Build history of the part. All positions in model axes, mm. A direction names the side the tool comes from. Round coordinates to 2 decimals unless told otherwise and drop trailing zeros. Order: outer loops, then holes, each group sorted by start corner. A loop starts at its lowest first (then second) coordinate and runs counter-clockwise, first axis right, second up. Notation, with made-up numbers: (49.25, 88) - (57.25, 88) arc R11 ccw to (57.25, 93) - close; hole circle Ø11 at (-17, 44). An arc over 180 degrees is marked (long way). One line per question, with ' | ' between items. Start each with the question number.
Autodesk Inventor part; units mm, degrees
ref_plane "YZ Plane" through (0, 0, 0) normal (1, 0, 0) x (0, 1, 0)
ref_plane "XZ Plane" through (0, 0, 0) normal (0, 1, 0) x (-1, 0, 0)
ref_plane "XY Plane" through (0, 0, 0) normal (0, 0, 1) x (1, 0, 0)
sketch "スケッチ1" plane through (0, 0, 0) normal (0, 1, 0) x (-1, 0, 0)
  line L0 (-15, -7.5) -> (15, -7.5)
  line L1 (15, -7.5) -> (15, 7.5)
  line L2 (15, 7.5) -> (-15, 7.5)
  line L3 (-15, 7.5) -> (-15, -7.5)
  line L4 (-15, -7.5) -> (15, 7.5) construction
  line L5 (15, -7.5) -> (-15, 7.5) construction
  point P0 (0, 0)
  dimension "d0" = 30
  dimension "d1" = 15
extrude "押し出し1" add sketch "スケッチ1" along normal mid plane 10
sketch "スケッチ2" plane through (0, 0, 0) normal (0, 1, 0) x (-1, 0, 0)
  line L0 (15, 7.5) -> (-15, 7.5)
  line L1 (10, 7.5) -> (-15, 7.5)
  line L2 (-15, 7.5) -> (-15, 1.5)
  line L3 (-15, 1.5) -> (10, 1.5)
  line L4 (10, 1.5) -> (10, 7.5)
  point P0 (0, 0)
  dimension "d4" = 25
  dimension "d5" = 6
  dimension "d6" = 5
extrude "押し出し2" cut sketch "スケッチ2" along normal mid plane 10
sketch "スケッチ3" plane through (0, 0, 0) normal (0, 1, 0) x (-1, 0, 0)
  line L0 (15, -7.5) -> (-15, -7.5)
  line L1 (-15, -7.5) -> (10, -7.5)
  line L2 (10, -7.5) -> (10, -1.5)
  line L3 (10, -1.5) -> (-15, -1.5)
  line L4 (-15, -1.5) -> (-15, -7.5)
  point P0 (0, 0)
  dimension "d9" = 25
  dimension "d10" = 6
extrude "押し出し3" cut sketch "スケッチ3" along normal mid plane 10
sketch "スケッチ4" plane through (0, 0, 0) normal (1, 0, 0) x (0, 1, 0)
  line L0 (2, 7.5) -> (-2, 7.5)
  line L1 (-2, 7.5) -> (-2, 2.5)
  line L2 (-2, 2.5) -> (2, 2.5)
  line L3 (2, 2.5) -> (2, 7.5)
  point P0 (0, 0)
  dimension "d13" = 4
  dimension "d14" = 5
  dimension "d15" = 2
  dimension "d16" = 7.5
extrude "押し出し4" cut sketch "スケッチ4" against normal blind 15
sketch "スケッチ6" plane through (0, 5, 0) normal (0, 1, 0) x (1, 0, 0)
  circle A0 centre (-12.5, -5) radius 1.25
  line L0 (-15, -7.5) -> (-10, -7.5)
  point P0 (0, 0)
  dimension "d23" = 2.5
  dimension "d24" = 2.5
extrude "押し出し5" cut sketch "スケッチ6" against normal blind 15
sketch "スケッチ7" plane through (0, 5, 0) normal (0, 1, 0) x (1, 0, 0)
  circle A0 centre (-12.5, 5) radius 1.25
  line L0 (-10, 7.5) -> (-15, 7.5)
  line L1 (-15, 7.5) -> (-15, -7.5)
  point P0 (0, 0)
  dimension "d27" = 2.5
  dimension "d28" = 2.5
extrude "押し出し6" cut sketch "スケッチ7" against normal blind 15
sketch "スケッチ8" plane through (-10, -5, -1.5) normal (1, 0, 0) x (0, 0, -1)
  line L0 (1, 7) -> (6, 7)
  line L1 (6, 7) -> (6, 3)
  line L2 (6, 3) -> (1, 3)
  line L3 (1, 3) -> (1, 7)
  point P0 (-1.5, 5)
  dimension "d32" = 5
  dimension "d33" = 4
  dimension "d34" = 7.5
  dimension "d35" = 2
extrude "押し出し7" cut sketch "スケッチ8" against normal blind 15
properties part number "promo_hold"
Item 1: Slice it at A-A (z = 5). Write the cut outline in (x, y), plus the area to 3 significant figures.
Item 2: Slice it at D-D (z = -3). Write the cut outline in (x, y).
Item 3: Pull direction X, two halves, no side cores. Call faces 1 (the face through (15, 0, 0)), 2 (the face through (-11, -2, 6)), 3 (the face through (-13.49, -3.48, 5.76)): released by +X, released by -X, zero draft, split by the parting line, or undercut.
Item 4: Wall check: line 1 along Z through (x, y) = (-12.5, 2.9); line 2 along X through (y, z) = (-4.4, -5); line 3 along Y through (x, z) = (-10.5, 6.25). Give the ranges that are in metal, low to high. Write a range as [from, to].
Item 5: Pin check, flat tips, straight feed: pin 1 (1 mm diameter, centred on x = 9, y = 1, fed in from -Z); pin 2 (4 mm diameter, centred on x = -12, z = -4, fed in from +Y); pin 3 (3 mm diameter, centred on x = -12.5, y = 0, fed in from -Z). Stop position of each tip, or through.
Item 6: Slice it at C-C (x = -12.5). Write the cut outline in (y, z), plus the area to 3 significant figures.
Item 7: Slice it at B-B (y = -3). Write the cut outline in (x, z).
Item 8: 3-axis set-ups, long thin cutter, end or side, ignore diameter. For faces 4 (the face through (-12, 0, 2.5)), 5 (the face through (3, 0, 1.5)), 6 (the face through (-12, 0, -2.5)), 7 (the face through (-10, -2.3, -4.5)): which of +Z, -Z, +X, -X, +Y, -Y reach the whole face in a straight line?
A:
1) outline: (-15, -5) - (-13.75, -5) - (-13.75, -2) - (-15, -2) - close; (-15, 2) - (-13.75, 2) - (-13.75, 5) - (-15, 5) - close; (-11.25, -5) - (-10, -5) - (-10, -2) - (-11.25, -2) - close; (-11.25, 2) - (-10, 2) - (-10, 5) - (-11.25, 5) - close | area: 15.0 mm^2
2) outline: (-15, -5) - (-10, -5) - (-10, -2) - (-15, -2) - close; (-15, 2) - (-10, 2) - (-10, 5) - (-15, 5) - close
3) face 1: released by +X | face 2: zero draft | face 3: undercut
4) line 1: [-7.5, -6.25], [-3.75, 3.75], [6.25, 7.5] | line 2: [-15, -13.75], [-11.25, -10] | line 3: [-5, -2], [2, 5]
5) pin 1: z = -1.5 | pin 2: y = 5 | pin 3: z = -2.5
6) outline: (-5, -7.5) - (-2, -7.5) - (-2, -6.25) - (-5, -6.25) - close; (-5, -3.75) - (-2, -3.75) - (-2, -2.5) - (2, -2.5) - (2, -3.75) - (5, -3.75) - (5, 3.75) - (2, 3.75) - (2, 2.5) - (-2, 2.5) - (-2, 3.75) - (-5, 3.75) - close; (-5, 6.25) - (-2, 6.25) - (-2, 7.5) - (-5, 7.5) - close; (2, -7.5) - (5, -7.5) - (5, -6.25) - (2, -6.25) - close; (2, 6.25) - (5, 6.25) - (5, 7.5) - (2, 7.5) - close | area: 80.0 mm^2
7) outline: (-15, -7.5) - (-10, -7.5) - (-10, -1.5) - (15, -1.5) - (15, 1.5) - (-10, 1.5) - (-10, 7.5) - (-15, 7.5) - close; hole circle Ø2.5 at (-12.5, -5); hole circle Ø2.5 at (-12.5, 5)
8) face 4: +Z, +X, -X | face 5: +Z, +X, +Y, -Y | face 6: -Z, +X, -X | face 7: -Z, +X, +Y, -Y
